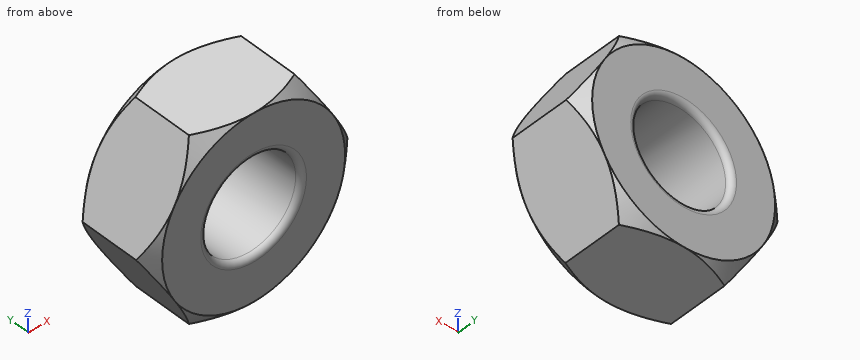
```python
from build123d import *

# Parameters (mm, degrees)
SALIENTE_EXTRUIR1_DEPTH = 15
CROQUIS2_OUTSIDE_W      = 81.348
CROQUIS2_OUTSIDE_H      = 76.398
CROQUIS2_OUTSIDE_R      = 16
CORTAR_EXTRUIR1_DEPTH   = 15
CORTAR_EXTRUIR1_TAPER   = 47
CROQUIS3_OUTSIDE_W      = 81.348
CROQUIS3_OUTSIDE_H      = 76.398
CROQUIS3_OUTSIDE_R      = 16
CORTAR_EXTRUIR2_DEPTH   = 15
CORTAR_EXTRUIR2_TAPER   = 47
CROQUIS4_R              = 8.25
CORTAR_EXTRUIR3_DEPTH   = 15
REDONDEO1_R             = 1


with BuildPart() as part:
    # Croquis1 → Saliente-Extruir1 (new body)
    with BuildSketch(Plane(origin=(0, 0, 0), x_dir=(1, 0, 0), z_dir=(0, 1, 0))):
        Polygon((-9.237604307, -16), (9.237604307, -16), (18.475208614, 0), (9.237604307, 16), (-9.237604307, 16), (-18.475208614, 0), align=None)
    extrude(amount=-SALIENTE_EXTRUIR1_DEPTH)

    # Croquis2 outside → Cortar-Extruir1 (cut)
    with BuildSketch(Plane(origin=(0, 0, 0), x_dir=(1, 0, 0), z_dir=(0, 1, 0))):
        Rectangle(CROQUIS2_OUTSIDE_W, CROQUIS2_OUTSIDE_H)
        Circle(CROQUIS2_OUTSIDE_R, mode=Mode.SUBTRACT)
    extrude(amount=-CORTAR_EXTRUIR1_DEPTH, taper=CORTAR_EXTRUIR1_TAPER, mode=Mode.SUBTRACT)

    # Croquis3 outside → Cortar-Extruir2 (cut)
    with BuildSketch(Plane.XZ.offset(15)):
        Rectangle(CROQUIS3_OUTSIDE_W, CROQUIS3_OUTSIDE_H)
        Circle(CROQUIS3_OUTSIDE_R, mode=Mode.SUBTRACT)
    extrude(amount=-CORTAR_EXTRUIR2_DEPTH, taper=CORTAR_EXTRUIR2_TAPER, mode=Mode.SUBTRACT)

    # Croquis4 → Cortar-Extruir3 (cut)
    with BuildSketch(Plane(origin=(0, 0, 0), x_dir=(1, 0, 0), z_dir=(0, 1, 0))):
        Circle(CROQUIS4_R)
    extrude(amount=-CORTAR_EXTRUIR3_DEPTH, mode=Mode.SUBTRACT)

    # Redondeo1
    redondeo1_edges = [part.edges().sort_by_distance(p)[0] for p in [
        (-8.25, -15, 0),
        (-8.25, 0, 0),
    ]]
    fillet(redondeo1_edges, radius=REDONDEO1_R)


solid = part.part
```
Geometry: final body of the model. Coordinates: model frame, mm. Round coordinates to 2 decimals unless told otherwise and drop trailing zeros. Order: outer loops, then holes, each group sorted by start corner. A loop starts at its lowest first (then second) coordinate and runs counter-clockwise, first axis right, second up. Notation, with made-up numbers: (88.5, 54.25) - (119.5, 54.25) arc R28 ccw to (119.5, 75.25) - close; hole circle Ø6 at (-5.5, 48). An arc over 180 degrees is marked (long way). Use CSV: the item, a comma, the result in double quotes. Start each with the question number.
Q1. Material intervals for line 1 along X through (y, z) = (-4, 0); line 2 along X through (y, z) = (-13.25, 6.5); line 3 along Z through (x, y) = (-3, -5), sorted ascending. Write a range as from..to.
Q2. Section query B-B (y = -13.5). Return loops of the section in (x, z), and give its area (3 significant figures).
Q3. Section query A-A (y = -3.75). Return loops of the section in (x, z).
Q4. First-contact query: pin 1 (3 mm diameter, centred on x = -13.5, y = -4, fed in from -Z); pin 2 (5 mm diameter, centred on x = 13, y = -2, fed in from -Z). Flat tips, straight axial feed; report the tip coordinate or a pass-through.
Result set:
1,line 1,"x = -18.48..-8.25, 8.25..18.48"
1,line 2,"x = -14.72..-5.08, 5.08..14.72"
1,line 3,"z = -16..-7.69, 7.69..16"
2,outline,"(-17.53, -1.63) - (-10.18, -14.37) arc R17.61 ccw to (-7.35, -16) - (7.35, -16) arc R17.61 ccw to (10.18, -14.37) - (17.53, -1.63) arc R17.61 ccw to (17.53, 1.63) - (10.18, 14.37) arc R17.61 ccw to (7.35, 16) - (-7.35, 16) arc R17.61 ccw to (-10.18, 14.37) - (-17.53, 1.63) arc R17.61 ccw to start; hole circle Ø16.5 at (0, 0)"
2,area,"665 mm2"
3,outline,"(-18.48, 0) - (-9.24, -16) - (9.24, -16) - (18.48, 0) - (9.24, 16) - (-9.24, 16) - close; hole circle Ø16.5 at (0, 0)"
4,pin 1,"stops at z = -11.22"
4,pin 2,"stops at z = -13.81"
